```python
from build123d import *

# Parameters (mm, degrees)
SKETCH1_W                = 5
SKETCH1_H                = 60
BOSS_EXTRUDE1_DEPTH      = 3
SKETCH2_R                = 1.5
BOSS_EXTRUDE2_DEPTH      = 10
FILLET1_R                = 1.5
BOSS_EXTRUDE3_DEPTH      = 10
BOSS_EXTRUDE3_DEPTH_BACK = 10
SKETCH3_R                = 1.5
FILLET2_R                = 1.5


with BuildPart() as part:
    # Sketch1 → Boss-Extrude1 (new body)
    with BuildSketch(Plane.XY):
        Rectangle(SKETCH1_W, SKETCH1_H)
    extrude(amount=BOSS_EXTRUDE1_DEPTH)

    # Sketch2 → Boss-Extrude2 (add)
    with BuildSketch(Plane(origin=(2.5, 0, 0), x_dir=(0, 0, -1), z_dir=(1, 0, 0))):
        with Locations(Location((-1.5, 28.5, 0), (0, 0, 90))):
            Circle(SKETCH2_R)
    extrude(amount=BOSS_EXTRUDE2_DEPTH)

    # Fillet1
    fillet1_edges = [part.edges().sort_by_distance(p)[0] for p in [
        (0, 30, 3),
        (0, 30, 0),
    ]]
    fillet(fillet1_edges, radius=FILLET1_R - 0.0001)  # a hair under: the kernel refuses the full size

    # Sketch3 → Boss-Extrude3 (add, two sides: drawn at the far end of the back side and taken through both)
    with BuildSketch(Plane.ZY.offset(-BOSS_EXTRUDE3_DEPTH_BACK)):
        with Locations(Location((1.5, -28.5, 0), (0, 0, 270))):
            Circle(SKETCH3_R)
    extrude(amount=BOSS_EXTRUDE3_DEPTH + BOSS_EXTRUDE3_DEPTH_BACK)

    # Fillet2
    fillet2_edges = [part.edges().sort_by_distance(p)[0] for p in [
        (0, -30, 3),
        (0, -30, 0),
    ]]
    fillet(fillet2_edges, radius=FILLET2_R - 0.0001)  # a hair under: the kernel refuses the full size


solid = part.part
```
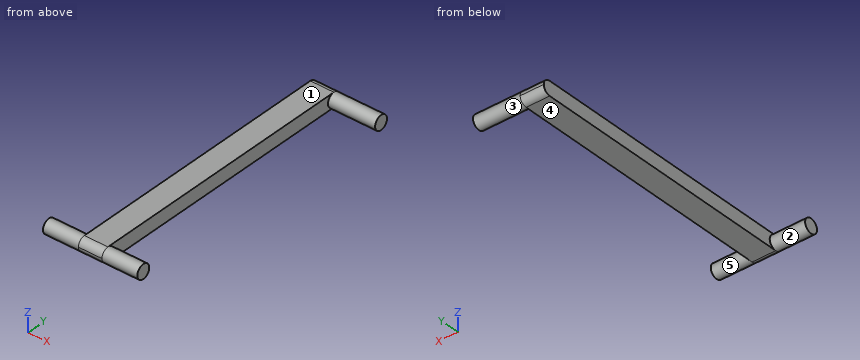
Here's how the part is built. I have some questions about the finished solid (model axes, mm). Face numbers are marked on the shaded views. A direction names the side the tool comes from. Give positions to 0.01 mm unless a question says otherwise; leave off trailing zeros. Write each loop counter-clockwise with the first axis right and the second up, starting at its lowest first coordinate (ties: lowest second). Pieces come first, ordered by that corner, then holes.
(1) Will these pins go through, and if not, where does the flat tip stop? pin 1 (1 mm diameter, centred on y = 3.5, z = 2, fed in from -X); pin 2 (1.2 mm diameter, centred on y = -29, z = 2.5, fed in from +X); pin 3 (1 mm diameter, centred on x = 8, z = 0.5, fed in from -Y).
Output values:
pin 1: stops at x = -2.5
pin 2: stops at x = 10
pin 3: stops at y = -29.91
(2) On a 3-axis mill with a long thin cutter (end or side, diameter ignored), from which of +Z, -Z, +X, -X, +Y, -Y can I reach the whole of each face in a straight line? I mean the marked faces 4 and 5. Say none if no direction works.
Output values:
face 4: -Z, +X, -X, +Y, -Y
face 5: +X
(3) Thinking about a two-plate mould opening in Y: for the marked faces 1, 2 and 3, which applies, pulls with the +Y half, pulls with the -Y half, needs draft (parallel to the pull), parting line crosses it, or undercut?
Output values:
face 1: needs draft
face 2: parting line crosses it
face 3: undercut
(4) Imagine slicing it at D-D, the plane x = -7. Write out the boundary of the cut face in (y, z), and give its area (3 significant figures).
Output values:
outline: circle Ø3 at (-28.5, 1.5)
area: 7.07 mm2
(5) Imagine slicing it at B-B, the plane x = 7.75. Write out the boundary of the cut face in (y, z), and give its area (3 significant figures).
Output values:
outline: circle Ø3 at (-28.5, 1.5); circle Ø3 at (28.5, 1.5)
area: 14.1 mm2
(6) Imagine slicing it at C-C, the plane y = 16. Write out the boundary of the cut face in (x, z), and give its area (3 significant figures).
Output values:
outline: (-2.5, 0) - (2.5, 0) - (2.5, 3) - (-2.5, 3) - close
area: 15.0 mm2
(7) If I drill on L1, parallel to X at y = -20.5, z = 2.05; L2, parallel to Y at x = -1.5, z = 1.7; L3, parallel to Y at x = 3, z = 0.4, over which ranges is the centre line in solid material (lowest first)?
Output values:
L1: x = -2.5 to 2.5
L2: y = -29.99 to 29.99
L3: y = -29.52 to -27.48, 27.48 to 29.52
